The listing builds one solid part. Answer for the finished solid, in the listing's coordinates (mm). Coordinates: 2 decimals unless noted, no trailing zeros.
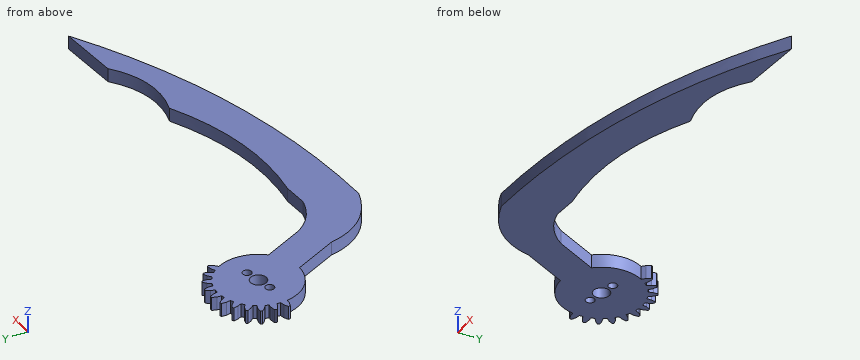
from build123d import *

# Parameters (mm, degrees)
SKETCH1_W           = 150
SKETCH1_H           = 70
BOSS_EXTRUDE1_DEPTH = 4
SKETCH2_W           = 150
SKETCH2_H           = 70
SKETCH2_R           = 1.3
SKETCH2_R_2         = 2.4
CUT_EXTRUDE1_DEPTH  = 10


with BuildPart() as part:
    # Sketch1 → Boss-Extrude1 (new body)
    with BuildSketch(Plane.XY):
        Rectangle(SKETCH1_W, SKETCH1_H)
    extrude(amount=BOSS_EXTRUDE1_DEPTH)

    # Sketch2 → Cut-Extrude1 (cut)
    # profile 1 of 4: a face of its own
    with BuildSketch(Plane.XY.offset(4)):
        Rectangle(SKETCH2_W, SKETCH2_H)
        with BuildLine():
            add(Edge.make_bspline(
                [(25.943186653, -3.950471355), (27.846969269, -4.547232813), (31.287122421, -5.290525852), (36.735640075, -5.338112806), (41.143250704, -4.366496225), (45.771671446, -2.369991596), (48.378055128, -0.634767364), (49.984542654, 0.667670418)],
                knots=[0, 0, 0, 0, 0.234141345, 0.410073985, 0.635494837, 0.757255977, 1, 1, 1, 1], degree=3))
            Line((49.984542654, 0.667670418), (68.368403063, 1.920292741))
            add(Edge.make_bspline(
                [(-33.004955139, -26.618623378), (-30.294523128, -26.574879913), (-25.880509709, -26.423954366), (-19.54201722, -26.014521717), (-14.319937046, -25.543432562), (-8.998131049, -24.92772797), (-2.890101028, -24.067514059), (4.364427962, -22.796901426), (11.870157255, -21.159659498), (19.827939937, -19.110263295), (26.884456831, -16.979260605), (34.037553038, -14.503385048), (39.936366025, -12.243402206), (45.782494162, -9.778756125), (51.423398212, -7.197801789), (59.009760326, -3.437427178), (64.682537278, -0.280517491), (68.368403063, 1.920292741)],
                knots=[0, 0, 0, 0, 0.076324938, 0.124331496, 0.178823517, 0.223936737, 0.275160112, 0.352480577, 0.431247301, 0.491394905, 0.583819579, 0.638693956, 0.704497251, 0.761639539, 0.81730198, 0.879134072, 1, 1, 1, 1], degree=3))
            add(Edge.make_bspline(
                [(-49.535748672, -9.096126268), (-49.339830369, -10.137896023), (-48.797352048, -12.328019472), (-47.539705157, -15.420109206), (-45.707187417, -18.401147763), (-43.54343584, -20.831673927), (-40.91315221, -22.974076428), (-37.51630052, -25.005074849), (-34.707117005, -26.096270898), (-33.004955139, -26.618623378)],
                knots=[0, 0, 0, 0, 0.124884489, 0.26543712, 0.391415345, 0.535530604, 0.646519487, 0.79009791, 1, 1, 1, 1], degree=3))
            Line((-49.535748672, -9.096126268), (-55.868573385, 3.961128214))
            ThreePointArc((-55.868573385, 3.961128214), (-63.649841308, 6.972432766), (-67.628790007, 14.306193932))
            Line((-67.628790007, 14.306193932), (-68.970840738, 14.428927947))
            Line((-68.970840738, 14.428927947), (-70.240707474, 14.880151039))
            Line((-70.240707474, 14.880151039), (-70.277437725, 15.5032436))
            Line((-70.277437725, 15.5032436), (-69.069379214, 16.10053619))
            Line((-69.069379214, 16.10053619), (-67.751042994, 16.380095513))
            Line((-67.751042994, 16.380095513), (-67.679030495, 17.409843403))
            Line((-67.679030495, 17.409843403), (-68.386470931, 17.681135001))
            Line((-68.386470931, 17.681135001), (-69.26282403, 18.111750468))
            Line((-69.26282403, 18.111750468), (-70.047304849, 18.693140424))
            Line((-70.047304849, 18.693140424), (-69.921515326, 19.304508109))
            Line((-69.921515326, 19.304508109), (-69.22879013, 19.48592239))
            Line((-69.22879013, 19.48592239), (-68.242063209, 19.582780663))
            Line((-68.242063209, 19.582780663), (-67.254259433, 19.497602945))
            Line((-67.254259433, 19.497602945), (-66.898609662, 20.523128894))
            Line((-66.898609662, 20.523128894), (-67.999492681, 21.300445035))
            Line((-67.999492681, 21.300445035), (-68.873617988, 22.326149063))
            Line((-68.873617988, 22.326149063), (-68.593881038, 22.884128176))
            Line((-68.593881038, 22.884128176), (-67.249025383, 22.797369477))
            Line((-67.249025383, 22.797369477), (-65.967533065, 22.380306842))
            Line((-65.967533065, 22.380306842), (-65.358576119, 23.278839907))
            Line((-65.358576119, 23.278839907), (-66.220763237, 24.314599134))
            Line((-66.220763237, 24.314599134), (-66.799631709, 25.531593422))
            Line((-66.799631709, 25.531593422), (-66.385010944, 25.998158608))
            Line((-66.385010944, 25.998158608), (-65.108434938, 25.566281883))
            Line((-65.108434938, 25.566281883), (-63.978552164, 24.831755694))
            Line((-63.978552164, 24.831755694), (-63.157787454, 25.542062333))
            Line((-63.157787454, 25.542062333), (-63.722522044, 26.765679367))
            Line((-63.722522044, 26.765679367), (-63.966684751, 28.091027765))
            Line((-63.966684751, 28.091027765), (-63.44543589, 28.434383377))
            Line((-63.44543589, 28.434383377), (-62.324136078, 27.686820312))
            Line((-62.324136078, 27.686820312), (-61.422862493, 26.684887316))
            Line((-61.422862493, 26.684887316), (-60.446223776, 27.158561304))
            Line((-60.446223776, 27.158561304), (-60.675020109, 28.486648666))
            Line((-60.675020109, 28.486648666), (-60.567837768, 29.830030872))
            Line((-60.567837768, 29.830030872), (-59.975483059, 30.026777792))
            Line((-59.975483059, 30.026777792), (-59.08587417, 29.014473574))
            Line((-59.08587417, 29.014473574), (-58.474630079, 27.813413848))
            Line((-58.474630079, 27.813413848), (-57.40867367, 28.018175086))
            Line((-57.40867367, 28.018175086), (-57.285939655, 29.360225818))
            Line((-57.285939655, 29.360225818), (-56.834716563, 30.630092553))
            Line((-56.834716563, 30.630092553), (-56.211624002, 30.666822805))
            Line((-56.211624002, 30.666822805), (-55.614331412, 29.458764294))
            Line((-55.614331412, 29.458764294), (-55.334772089, 28.140428074))
            Line((-55.334772089, 28.140428074), (-54.252141156, 28.062322422))
            Line((-54.252141156, 28.062322422), (-53.786240912, 29.326877983))
            Line((-53.786240912, 29.326877983), (-53.021727178, 30.436689929))
            Line((-53.021727178, 30.436689929), (-52.410359493, 30.310900406))
            Line((-52.410359493, 30.310900406), (-52.146087704, 28.989414792))
            Line((-52.146087704, 28.989414792), (-52.217264657, 27.643644513))
            Line((-52.217264657, 27.643644513), (-51.191738708, 27.287994742))
            Line((-51.191738708, 27.287994742), (-50.414422567, 28.388877761))
            Line((-50.414422567, 28.388877761), (-49.388718539, 29.263003067))
            Line((-49.388718539, 29.263003067), (-48.830739426, 28.983266117))
            Line((-48.830739426, 28.983266117), (-48.917498125, 27.638410463))
            Line((-48.917498125, 27.638410463), (-49.33456076, 26.356918144))
            Line((-49.33456076, 26.356918144), (-48.436027695, 25.747961199))
            Line((-48.436027695, 25.747961199), (-47.400268467, 26.610148317))
            Line((-47.400268467, 26.610148317), (-46.18327418, 27.189016789))
            Line((-46.18327418, 27.189016789), (-45.716708994, 26.774396023))
            Line((-45.716708994, 26.774396023), (-46.148585719, 25.497820017))
            Line((-46.148585719, 25.497820017), (-46.883111907, 24.367937244))
            Line((-46.883111907, 24.367937244), (-46.172805269, 23.547172533))
            Line((-46.172805269, 23.547172533), (-45.286864939, 23.992280694))
            Line((-45.286864939, 23.992280694), (-44.334478382, 24.26790977))
            Line((-44.334478382, 24.26790977), (-43.623839837, 24.356069831))
            Line((-43.623839837, 24.356069831), (-43.280484225, 23.83482097))
            Line((-43.280484225, 23.83482097), (-44.02804729, 22.713521158))
            Line((-44.02804729, 22.713521158), (-45.029980286, 21.812247573))
            ThreePointArc((-45.029980286, 21.812247573), (-43.655526666, 14.616368623), (-46.687860181, 7.947429421))
            Line((-46.687860181, 7.947429421), (-40.625414849, -4.552346756))
            add(Edge.make_bspline(
                [(-40.625414849, -4.552346756), (-39.969724138, -5.518615353), (-38.642033006, -7.159979255), (-36.383256782, -9.119344727), (-34.181437855, -10.482492748), (-31.814725419, -11.517519607), (-30.173224961, -11.982812896), (-29.2632985, -12.178103902)],
                knots=[0, 0, 0, 0, 0.249608299, 0.449336056, 0.636249607, 0.801036873, 1, 1, 1, 1], degree=3))
            Line((-29.2632985, -12.178103902), (-21.905328426, -11.80268597))
            add(Edge.make_bspline(
                [(-21.905328426, -11.80268597), (-20.310852996, -12.055092712), (-17.169889797, -12.459787879), (-12.483928013, -12.782767249), (-8.045859096, -12.82243272), (-3.649062985, -12.608578219), (1.283313279, -12.08050338), (5.938716144, -11.233581759), (10.05540984, -10.206537199), (13.081948519, -9.312895411), (16.474512339, -8.1639354), (20.793643696, -6.464082533), (24.086370836, -4.909244471), (25.943186653, -3.950471355)],
                knots=[0, 0, 0, 0, 0.098157301, 0.192485818, 0.285432427, 0.367865586, 0.460021268, 0.586889267, 0.655198895, 0.717943591, 0.778718956, 0.872950297, 1, 1, 1, 1], degree=3))
        make_face(mode=Mode.SUBTRACT)
    # profile 2 of 4: a face of its own
    with BuildSketch(Plane.XY.offset(4)):
        with Locations((-60.081947299, 15.203234123)):
            Circle(SKETCH2_R)
    # profile 3 of 4: a face of its own
    with BuildSketch(Plane.XY.offset(4)):
        with Locations((-51.243535224, 16.901018558)):
            Circle(SKETCH2_R)
    # profile 4 of 4: a face of its own
    with BuildSketch(Plane.XY.offset(4)):
        with Locations((-55.662741261, 16.052126341)):
            Circle(SKETCH2_R_2)
    extrude(amount=-CUT_EXTRUDE1_DEPTH, mode=Mode.SUBTRACT)


solid = part.part
1. Section A-A on z = 1.05 is taken. State how many separate pieces and enclosed holes the cut face has, then the cut area to 3 significant figures.
Results found:
separate pieces: 1
enclosed holes: 3
area: 1,880 mm2
2. Flat-ended cylindrical pins translate along their axes: P1, Ø2, axis at y = -1.5, z = 3, coming from the -X side; P2, Ø2, axis at x = 16.5, z = 2.5, coming from the +Y side; P3, Ø2.5, axis at x = -60.08, y = 15.2, coming from the -Z side; P4, Ø1, axis at x = -20.5, z = 2, coming from the -Y side. Find the tip coordinate at first contact, or state that the pin passes through.
Results found:
P1: stops at x = -53.7
P2: stops at y = -7.75
P3: passes through
P4: stops at y = -26.1
3. Find the intervals of material crossed by L1, parallel to X at y = 28.5, z = 2.55; L2, parallel to X at y = -0.5, z = 0.25; L3, parallel to X at y = 10, z = 3.8, in increasing order.
Results found:
L1: x = -60.67 to -58.82, -57.36 to -55.41, -54.09 to -52.17, -50.28 to -48.86
L2: x = -53.7 to -42.59, 48.45 to 64.21
L3: x = -66.13 to -45.19
